The model under review builds one solid part; all positions refer to its coordinate system, in mm. Coordinates: 2 decimals unless noted, no trailing zeros. Write each loop counter-clockwise with the first axis right and the second up, starting at its lowest first coordinate (ties: lowest second). Pieces come first, ordered by that corner, then holes. Notation, with made-up numbers: (60, 43.25) - (71, 43.25) arc R16 cw to (71, 52.25) - close; hole circle Ø1 at (9, 72.5). An arc over 180 degrees is marked (long way). Put each result on its own line as item: value. Start each with the question number.
Item 1: For pin 1 (0.6 mm diameter, centred on x = -42.5, z = 1.5, fed in from -Y), flat-tipped, find the tip position at first contact; note if it passes through.
Item 2: Consider section C-C on z = 0.3. Give the boundary of the cut face in (x, y).
Item 3: Consider section D-D on x = -51.5. Give the boundary of the cut face in (y, z).
Item 4: To check wall thickness, follow L1, parallel to Y at x = 154.5, z = 1.1; L2, parallel to Y at x = -88, z = 0.4; L3, parallel to X at y = 11.5, z = 0.7. State the ranges of each line that lie inside material, in increasing order. Write a range as [from, to].
Item 5: Consider section A-A on y = 17. Give the boundary of the cut face in (x, z), then the cut area to 3 significant figures.
Item 6: Mouldability with a two-part tool opening along X and no side actions: class faces 1 (the face through (57.4, -126.22, 0.99)), 2 (the face through (188.88, 114.87, 0.99)), 3 (the face through (129.524, -140.901, 1.014)) as pulls with the +X half, pulls with the -X half, needs draft (parallel to the pull), parting line crosses it, or undercut.
Item 7: Consider section B-B on x = 154.5. Give the boundary of the cut face in (y, z), then the cut area to 3 significant figures.
Autodesk Inventor part; units mm, degrees
ref_plane "YZ Plane" through (0, 0, 0) normal (1, 0, 0) x (0, 1, 0)
ref_plane "XZ Plane" through (0, 0, 0) normal (0, 1, 0) x (-1, 0, 0)
ref_plane "XY Plane" through (0, 0, 0) normal (0, 0, 1) x (1, 0, 0)
sketch "Эскиз1" plane through (0, 0, 0) normal (0, 0, 1) x (1, 0, 0)
  line L0 (-166.5, -124) -> (46.0736, -124)
  line L1 (198.5, -124) -> (198.5, 92)
  line L2 (166.5, 124) -> (-166.5, 124)
  line L3 (-198.5, 92) -> (-198.5, -92)
  line L4 (-198.5, -124) -> (198.5, 124) construction
  line L5 (198.5, -124) -> (-198.5, 124) construction
  arc A0 (-166.5, 124) -> (-198.5, 92) centre (-166.5, 92) ccw
  arc A1 (198.5, 92) -> (166.5, 124) centre (166.5, 92) ccw
  arc A2 (-198.5, -92) -> (-166.5, -124) centre (-166.5, -92) ccw
  line L6 (198.5, -124) -> (198.5, -162)
  line L7 (186.5, -174) -> (120.9264, -174)
  line L8 (99.7132, -165.2132) -> (67.2868, -132.7868)
  arc A3 (186.5, -174) -> (198.5, -162) centre (186.5, -162) ccw
  arc A4 (99.7132, -165.2132) -> (120.9264, -174) centre (120.9264, -144) ccw
  arc A5 (67.2868, -132.7868) -> (46.0736, -124) centre (46.0736, -154) ccw
  point P0 (0, 0)
  point P1 (198.5, -174)
  point P2 (108.5, -174)
  dimension "d2" = 397
  dimension "d3" = 248
  dimension "d4" = 32
  dimension "d5" = 298
  dimension "d6" = 12
  dimension "d7" = 50
  dimension "d8" = 90
  dimension "d9" = 135
  dimension "d10" = 30
extrude "Пластина1" add sketch "Эскиз1" along normal blind 2
sketch "Эскиз5" plane through (0, 0, 2) normal (0, 0, 1) x (1, 0, 0)
  line L0 (198.5, 92) -> (198.5, -162)
  arc A0 (198.5, 92) -> (166.5, 124) centre (166.5, 92) ccw
  line L1 (-166.5, 124) -> (166.5, 124)
  arc A1 (-166.5, 124) -> (-198.5, 92) centre (-166.5, 92) ccw
  line L2 (-198.5, -92) -> (-198.5, 92)
  arc A2 (-198.5, -92) -> (-166.5, -124) centre (-166.5, -92) ccw
  line L3 (46.0736, -124) -> (-166.5, -124)
  arc A3 (67.2868, -132.7868) -> (46.0736, -124) centre (46.0736, -154) ccw
  line L4 (99.7132, -165.2132) -> (67.2868, -132.7868)
  arc A4 (99.7132, -165.2132) -> (120.9264, -174) centre (120.9264, -144) ccw
  line L5 (186.5, -174) -> (120.9264, -174)
  arc A5 (186.5, -174) -> (198.5, -162) centre (186.5, -162) ccw
  circle A6 centre (154.5, -142) radius 25
  line L6 (-172, 97.5) -> (172, 97.5)
  line L7 (172, 97.5) -> (172, -94.5)
  line L8 (172, -94.5) -> (-172, -94.5)
  line L9 (-172, -94.5) -> (-172, 97.5)
  point P0 (0, 0)
  dimension "d57" = 50
  dimension "d58" = 26.5
  dimension "d59" = 26.5
  dimension "d60" = 26.5
  dimension "d61" = 29.5
  dimension "d62" = 44
  dimension "d63" = 32
extrude "Вырез4" cut sketch "Эскиз5" against normal blind 2 contours A6 | L6 L7 L8 L9
fillet "УглСкругление1" radius 6 4 edges at (-172, 97.5, 1) (172, 97.5, 1) (172, -94.5, 1) (-172, -94.5, 1)
equation "\"d59\" = d60"
equation "\"d64\" = Толщина"
equation "\"d12\" = Толщина"
equation "\"Радиус_гибки\" = Толщина"
equation "\"Ширина_просечки\" = Толщина"
equation "\"Глубина_просечки\" = 0.5 * Толщина"
equation "\"Размер_просечки\" = 4 * Толщина"
equation "\"Мин_остаток\" = 2 * Толщина"
equation "\"Радиус_перехода\" = Радиус_гибки"
equation "\"Радиус_Якоби\" = Радиус_гибки"
equation "\"Размер_зазора\" = Толщина"
properties part number "Стекло"
Report:
1. pin 1: y = -124
2. outline: (-198.5, -92) arc R32 ccw to (-166.5, -124) - (46.07, -124) arc R30 cw to (67.29, -132.79) - (99.71, -165.21) arc R30 ccw to (120.93, -174) - (186.5, -174) arc R12 ccw to (198.5, -162) - (198.5, 92) arc R32 ccw to (166.5, 124) - (-166.5, 124) arc R32 ccw to (-198.5, 92) - close; hole (-172, -88.5) arc R6 ccw to (-166, -94.5) - (166, -94.5) arc R6 ccw to (172, -88.5) - (172, 91.5) arc R6 ccw to (166, 97.5) - (-166, 97.5) arc R6 ccw to (-172, 91.5) - close; hole circle Ø50 at (154.5, -142)
3. outline: (-124, 0) - (-94.5, 0) - (-94.5, 2) - (-124, 2) - close; (97.5, 0) - (124, 0) - (124, 2) - (97.5, 2) - close
4. L1: [-174, -167], [-117, -94.5], [97.5, 124]
4. L2: [-124, -94.5], [97.5, 124]
4. L3: [-198.5, -172], [172, 198.5]
5. outline: (-198.5, 0) - (-172, 0) - (-172, 2) - (-198.5, 2) - close; (172, 0) - (198.5, 0) - (198.5, 2) - (172, 2) - close
5. area: 106 mm²
6. face 1: pulls with the -X half
6. face 2: pulls with the +X half
6. face 3: undercut
7. outline: (-174, 0) - (-167, 0) - (-167, 2) - (-174, 2) - close; (-117, 0) - (-94.5, 0) - (-94.5, 2) - (-117, 2) - close; (97.5, 0) - (124, 0) - (124, 2) - (97.5, 2) - close
7. area: 112 mm²
